from build123d import *

# Parameters (mm, degrees)
FILLET1_R   = 0.1
HEX_2_DEPTH = 1.1


with BuildPart() as part:
    # BodySke → BaseBody (revolve)
    with BuildSketch(Plane.XY):
        Polygon((0, 0), (0, 2.675), (0.685, 2.675), (1.86, 1.5), (24.7195, 1.5), (25, 1.2195), (25, 0), align=None)
    revolve(axis=Axis((0, 0, 0), (1, 0, 0)))

    # Fillet1
    fillet1_edges = [part.edges().sort_by_distance(p)[0] for p in [
        (1.86, -1.5, 0),
    ]]
    fillet(fillet1_edges, radius=FILLET1_R)

    # Sketch2 → PreBroach (revolve, cut)
    with BuildSketch(Plane.XY):
        Polygon((0, 1), (1.1, 1), (1.677350269, 0), (0, 0), align=None)
    revolve(axis=Axis((0, 0, 0), (1, 0, 0)), mode=Mode.SUBTRACT)

    # Sketch3 → Hex 2 (cut)
    with BuildSketch(Plane.ZY):
        Polygon((-1, -0.577350269), (-1, 0.577350269), (0, 1.154700538), (1, 0.577350269), (1, -0.577350269), (0, -1.154700538), align=None)
    extrude(amount=-HEX_2_DEPTH, mode=Mode.SUBTRACT)


solid = part.part
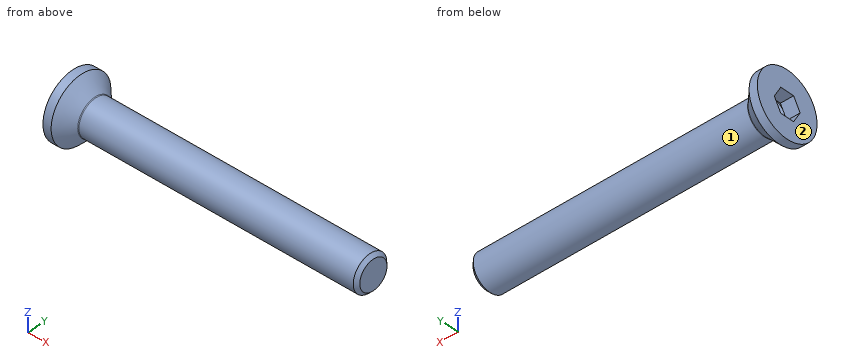
Model file for the job. Use its own axes, mm. Face numbers are marked on the shaded views. A direction names the side the tool comes from. Give positions to 0.01 mm unless a question says otherwise; leave off trailing zeros. Order: outer loops, then holes, each group sorted by start corner. A loop starts at its lowest first (then second) coordinate and runs counter-clockwise, first axis right, second up. Notation, with made-up numbers: (20, 75.25) - (33, 75.25) arc R9 cw to (33, 87.25) - close; hole circle Ø3 at (-3, 73). An arc over 180 degrees is marked (long way). One line per item, written item: value.
Item 1: Pin check, flat tips, straight feed: pin 1 Ø1 at (x, z) = (11.5, 0) entering from +Y; pin 2 Ø1 at (x, z) = (6.5, -1) entering from +Y. Stop position of each tip, or through.
Response values:
pin 1: y = 1.5
pin 2: y = 1.41
Item 2: Wall check: line 1 (Y direction, x = 2, z = -0.1); line 2 (X direction, y = 0.8, z = 1.85); line 3 (Y direction, x = 5.75, z = 0.75). Give the ranges that are in metal, low to high.
Response values:
line 1: -1.5 to 1.5
line 2: 0 to 1.34
line 3: -1.3 to 1.3
Item 3: Tool access for the marked faces 1 and 2: list every direction of +Z, -Z, +X, -X, +Y, -Y with a clear straight run to the whole face (end or side of a thin tool).
Response values:
face 1: +X
face 2: +Z, -Z, -X, +Y, -Y
Item 4: Slice it at A-A (x = 5.5). List the corners of the cut face in (y, z).
Response values:
outline: circle Ø3 at (0, 0)
